Here's how the part is built. I have some questions about the finished solid (model axes, mm). A direction names the side the tool comes from. Round coordinates to 2 decimals unless told otherwise and drop trailing zeros. Loops run counter-clockwise (first coordinate to the right, second up) from the corner with the lowest first, then second, coordinate; pieces in that order, holes last. Notation, with made-up numbers: M 84.5,-35 L 112.5,-35 A23 cw 112.5,-17 Z; hole C 19,10.5 d1. An arc over 180 degrees is marked long. Use a Markdown table: item, result.
from build123d import *

# Parameters (mm, degrees)
SKETCH1_R                = 100
BOSS_EXTRUDE1_DEPTH      = 120
SKETCH2_R                = 160
BOSS_EXTRUDE3_DEPTH      = 16
SKETCH3_R                = 130
SKETCH3_R_2              = 75
BOSS_EXTRUDE4_DEPTH      = 90
BOSS_EXTRUDE5_REACH      = 402.125
BOSS_EXTRUDE5_END_RADIUS = 130
SKETCH4_W                = 220
SKETCH4_H                = 160
FILLET1_R                = 10


with BuildPart() as part:
    # Sketch1 → Boss-Extrude1 (new body)
    with BuildSketch(Plane(origin=(0, 0, 0), x_dir=(1, 0, 0), z_dir=(0, 1, 0))):
        with Locations(Location((0, 0, 0), (0, 0, 270))):
            Circle(SKETCH1_R)
    extrude(amount=BOSS_EXTRUDE1_DEPTH)

    # Sketch2 → Boss-Extrude3 (add)
    with BuildSketch(Plane(origin=(0, 120, 0), x_dir=(1, 0, 0), z_dir=(0, 1, 0))):
        with Locations(Location((0, 0, 0), (0, 0, 270))):
            Circle(SKETCH2_R)
    extrude(amount=BOSS_EXTRUDE3_DEPTH)



with BuildPart() as body_2:
    # Sketch3 → Boss-Extrude4 (new, symmetric)
    with BuildSketch(Plane.XY):
        with Locations(Location((0, 336, 0), (0, 0, 180))):
            Circle(SKETCH3_R)
        with Locations(Location((0, 336, 0), (0, 0, 180))):
            Circle(SKETCH3_R_2, mode=Mode.SUBTRACT)
    extrude(amount=BOSS_EXTRUDE4_DEPTH, both=True)


with BuildPart() as part_1:
    add(part.part)

    add(body_2.part)  # Boss-Extrude5 merges body 2
    # Boss-Extrude5: up to this cylinder (the profile starts outside it)
    boss_extrude5_end = Plane(origin=(0, 336, 0), z_dir=(0, 0, -1)) * Cylinder(BOSS_EXTRUDE5_END_RADIUS, 1065.25, mode=Mode.PRIVATE)
    # Sketch4 → Boss-Extrude5 (add, up to the surface)
    with BuildSketch(Plane(origin=(0, 136, 0), x_dir=(1, 0, 0), z_dir=(0, 1, 0)), mode=Mode.PRIVATE) as boss_extrude5_sk1:
        Rectangle(SKETCH4_W, SKETCH4_H)
    boss_extrude5_tool1 = extrude(boss_extrude5_sk1.sketch, amount=BOSS_EXTRUDE5_REACH, mode=Mode.PRIVATE) - boss_extrude5_end
    add(boss_extrude5_tool1.solids().sort_by_distance((0, 136, 0))[0])

    # Fillet1
    fillet1_edges = [part_1.edges().sort_by_distance(p)[0] for p in [
        (110, 201.358983849, -80),
        (110, 201.358983849, 80),
        (-110, 201.358983849, -80),
        (-110, 201.358983849, 80),
    ]]
    fillet(fillet1_edges, radius=FILLET1_R)


solid = part_1.part
1. We'd pull the mould along Y, two halves only. Please class faces 1 (the face through (1, 0, -1)), 2 (the face through (9.764, 261.638, -1.26)), 3 (the face through (30.04, 59.16, 95.38)), 4 (the face through (-1, 181, -80)): +Y half, -Y half, draft (parallel to the pull), parting line (faces both ways), or undercut.
Answer sheet:
| item | result |
|---|---|
| face 1 | -Y half |
| face 2 | undercut |
| face 3 | draft |
| face 4 | undercut |
2. Imagine slicing it at A-A, the plane x = 0. Write out the boundary of the cut face in (y, z), then the cut area to 3 significant figures.
Answer sheet:
| item | result |
|---|---|
| outline | M 0,-100 L 120,-100 L 120,-160 L 136,-160 L 136,-80 L 206,-80 L 206,-90 L 261,-90 L 261,90 L 206,90 L 206,80 L 136,80 L 136,160 L 120,160 L 120,100 L 0,100 Z; M 411,-90 L 466,-90 L 466,90 L 411,90 Z |
| area | 60,100 mm2 |
3. Which directions (+Z, -Z, +X, -X, +Y, -Y) give clear straight access to the entire face, cutting with the end or side of a thin tool? Please do faces 5 (the face through (-56, 392, -90)), 6 (the face through (73, 120, 69)), 7 (the face through (-107.15, 202.27, -76.99)), 8 (the face through (-107.15, 202.27, 76.99)), 9 (the face through (110, 200, 1)).
Answer sheet:
| item | result |
|---|---|
| face 5 | -Z, +X, -X, +Y |
| face 6 | -Y |
| face 7 | -Z, -X |
| face 8 | +Z, -X |
| face 9 | +Z, -Z, +X |
4. Imagine slicing it at B-B, the plane y = 336. Write out the boundary of the cut face in (x, z).
Answer sheet:
| item | result |
|---|---|
| outline | M -130,-90 L -75,-90 L -75,90 L -130,90 Z; M 75,-90 L 130,-90 L 130,90 L 75,90 Z |
5. Imagine slicing it at D-D, the plane x = 82.5. Write out the boundary of the cut face in (y, z), then the cut area to 3 significant figures.
Answer sheet:
| item | result |
|---|---|
| outline | M 0,-56.51 L 120,-56.51 L 120,-137.09 L 136,-137.09 L 136,-80 L 235.53,-80 L 235.53,-90 L 436.47,-90 L 436.47,90 L 235.53,90 L 235.53,80 L 136,80 L 136,137.09 L 120,137.09 L 120,56.51 L 0,56.51 Z |
| area | 70,000 mm2 |
6. Imagine slicing it at C-C, the plane z = 0. Write out the boundary of the cut face in (x, y), then the cut area to 3 significant figures.
Answer sheet:
| item | result |
|---|---|
| outline | M -160,120 L -100,120 L -100,0 L 100,0 L 100,120 L 160,120 L 160,136 L 110,136 L 110,266.72 A130 ccw long -110,266.72 L -110,136 L -160,136 Z; hole C 0,336 d150 |
| area | 83,900 mm2 |
7. For pin 1 Ø3 at (y, z) = (66, 37.5) entering from +X; pin 2 Ø8 at (x, y) = (-90.5, 107) entering from +Z; pin 3 Ø10 at (y, z) = (358, -36.5) entering from +X, each with a flat end and sliding along its axis, tell me the tip position at first contact or that it passes through.
Answer sheet:
| item | result |
|---|---|
| pin 1 | x = 93.3 |
| pin 2 | z = 50.18 |
| pin 3 | x = 128.88 |
8. I need wall thicknesses on probe 1 along Y at (x, z) = (0, -53); probe 2 along X at (y, z) = (336, -45); probe 3 along Y at (x, z) = (-108, -100). Which ranges of each line are inside material? Lowest first, please. Write a range as from..to.
Answer sheet:
| item | result |
|---|---|
| probe 1 | 0..261, 411..466 |
| probe 2 | -130..-75, 75..130 |
| probe 3 | 120..136 |
